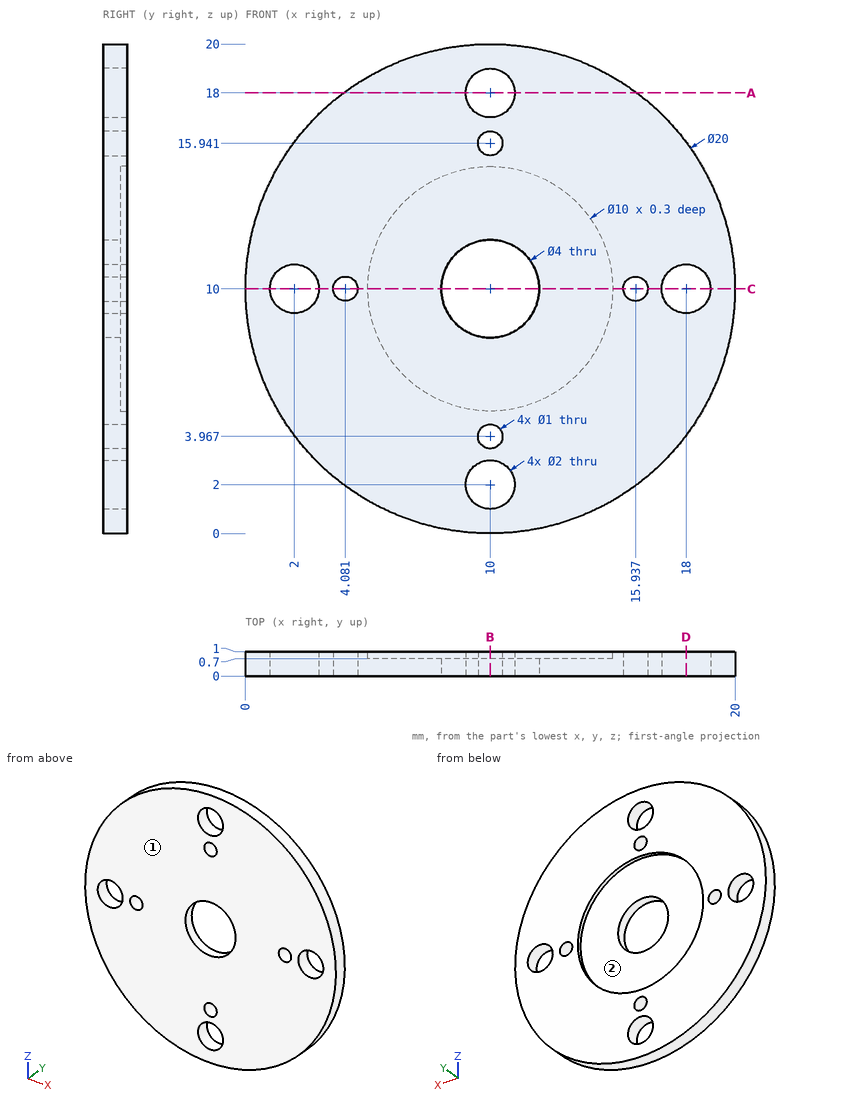
Geometry check sheet. Reference: drawing and pictorial views, mm from the part's lowest x, y, z. Round coordinates to 2 decimals unless told otherwise and drop trailing zeros. Write each loop counter-clockwise with the first axis right and the second up, starting at its lowest first coordinate (ties: lowest second). Pieces come first, ordered by that corner, then holes. Notation, with made-up numbers: (17, 60) -> (39, 60) arc R15 ccw to (39, 78) -> close; hole circle Ø6 at (-3.5, -8). An arc over 180 degrees is marked (long way). Put each result on its own line as item: value.
1) Release check for a two-part mould opening along Z. For the marked faces 1 and 2 record: pulls with the +Z half, pulls with the -Z half, needs draft (parallel to the pull), parting line crosses it, or undercut.
Recorded:
face 1: needs draft
face 2: undercut
2) Cross-section at C-C, the plane z = 10. Enter the section's corners in (x, y).
Recorded:
outline: (0, 0) -> (1, 0) -> (1, 1) -> (0, 1) -> close; (3, 0) -> (3.58, 0) -> (3.58, 1) -> (3, 1) -> close; (4.58, 0) -> (8, 0) -> (8, 0.7) -> (5, 0.7) -> (5, 1) -> (4.58, 1) -> close; (12, 0) -> (15.44, 0) -> (15.44, 1) -> (15, 1) -> (15, 0.7) -> (12, 0.7) -> close; (16.44, 0) -> (17, 0) -> (17, 1) -> (16.44, 1) -> close; (19, 0) -> (20, 0) -> (20, 1) -> (19, 1) -> close
3) Cross-section at A-A, the plane z = 18. Enter the section's corners in (x, y), plus the area to 3 significant figures.
Recorded:
outline: (4, 0) -> (9, 0) -> (9, 1) -> (4, 1) -> close; (11, 0) -> (16, 0) -> (16, 1) -> (11, 1) -> close
area: 10.0 mm2
4) Thickness scan on probe 1 along X at (y, z) = (0.3, 10); probe 2 along X at (y, z) = (0.85, 10); probe 3 along Y at (x, z) = (9, 14). Record the ranges inside material, lowest first. Write a range as from..to.
Recorded:
probe 1: x = 0..1, 3..3.58, 4.58..8, 12..15.44, 16.44..17, 19..20
probe 2: x = 0..1, 3..3.58, 4.58..5, 15..15.44, 16.44..17, 19..20
probe 3: y = 0..0.7
5) Cross-section at B-B, the plane x = 10. Enter the section's corners in (y, z).
Recorded:
outline: (0, 0) -> (1, 0) -> (1, 1) -> (0, 1) -> close; (0, 3) -> (1, 3) -> (1, 3.47) -> (0, 3.47) -> close; (0, 4.47) -> (1, 4.47) -> (1, 5) -> (0.7, 5) -> (0.7, 8) -> (0, 8) -> close; (0, 12) -> (0.7, 12) -> (0.7, 15) -> (1, 15) -> (1, 15.44) -> (0, 15.44) -> close; (0, 16.44) -> (1, 16.44) -> (1, 17) -> (0, 17) -> close; (0, 19) -> (1, 19) -> (1, 20) -> (0, 20) -> close
6) Depth check by flat-ended pin: P1, Ø1.6, axis at x = 2, z = 10, coming from the -Y side; P2, Ø9, axis at x = 10, z = 10, coming from the +Y side. Enter the tip coordinate at first touch or a pass-through.
Recorded:
P1: passes through
P2: stops at y = 0.7
7) Cross-section at D-D, the plane x = 18. Enter the section's corners in (y, z), plus the area to 3 significant figures.
Recorded:
outline: (0, 4) -> (1, 4) -> (1, 9) -> (0, 9) -> close; (0, 11) -> (1, 11) -> (1, 16) -> (0, 16) -> close
area: 10.0 mm2
